```python
from build123d import *

# Parameters (mm, degrees)
EXTRUDE_2_DEPTH     = 3
SKETCH_4_R          = 2.25
SKETCH_4_R_2        = 2.5
CUT_EXTRUDE_2_DEPTH = 96.402519291
SKETCH_6_R          = 3.5
CUT_EXTRUDE_3_DEPTH = 96.402519291
SKETCH_7_R          = 3.5
CUT_EXTRUDE_4_DEPTH = 96.402519291
CUT_EXTRUDE_5_DEPTH = 96.402519291


with BuildPart() as part:
    # 草图2 → 凸台-拉伸2 (new body)
    with BuildSketch(Plane(origin=(0, 0, 0), x_dir=(1, 0, 0), z_dir=(0, 1, 0))):
        with BuildLine():
            Line((-58.569449541, 23.337085947), (32.740581269, -53.879999426))
            ThreePointArc((32.740581269, -53.879999426), (53.033008589, -53.033008589), (53.879999426, -32.740581269))
            Line((53.879999426, -32.740581269), (-23.337085947, 58.569449541))
            ThreePointArc((-23.337085947, 58.569449541), (-60.104076401, 60.104076401), (-58.569449541, 23.337085947))
        make_face()
    extrude(amount=EXTRUDE_2_DEPTH)

    # 草图4 → 切除-拉伸2 (cut, through all)
    with BuildSketch(Plane(origin=(0, 3, 0), x_dir=(1, 0, 0), z_dir=(0, 1, 0))):
        with Locations(Location((-42.426406871, 42.426406871, 0), (0, 0, 270))):
            Circle(SKETCH_4_R)
        with Locations(Location((42.426406871, -42.426406871, 0), (0, 0, 270))):
            Circle(SKETCH_4_R_2)
    extrude(amount=-CUT_EXTRUDE_2_DEPTH, mode=Mode.SUBTRACT)

    # 草图6 → 切除-拉伸3 (cut, through all)
    with BuildSketch(Plane(origin=(0, 3, 0), x_dir=(1, 0, 0), z_dir=(0, 1, 0))):
        with Locations(Location((-42.426406871, 42.426406871, 0), (0, 0, 270))):
            Circle(SKETCH_6_R)
    extrude(amount=-CUT_EXTRUDE_3_DEPTH, mode=Mode.SUBTRACT)

    # 草图7 → 切除-拉伸4 (cut, through all)
    with BuildSketch(Plane(origin=(0, 3, 0), x_dir=(1, 0, 0), z_dir=(0, 1, 0))):
        with Locations(Location((42.426406871, -42.426406871, 0), (0, 0, 270))):
            Circle(SKETCH_7_R)
    extrude(amount=-CUT_EXTRUDE_4_DEPTH, mode=Mode.SUBTRACT)

    # 草图8 → 切除-拉伸5 (cut, through all)
    with BuildSketch(Plane(origin=(0, 3, 0), x_dir=(1, 0, 0), z_dir=(0, 1, 0))):
        Polygon((33.626672858, -22.564710472), (-15.702999665, 25.870376375), (-26.891422763, 12.98046534), (25.218843822, -32.251166492), align=None)
    extrude(amount=-CUT_EXTRUDE_5_DEPTH, mode=Mode.SUBTRACT)


solid = part.part
```
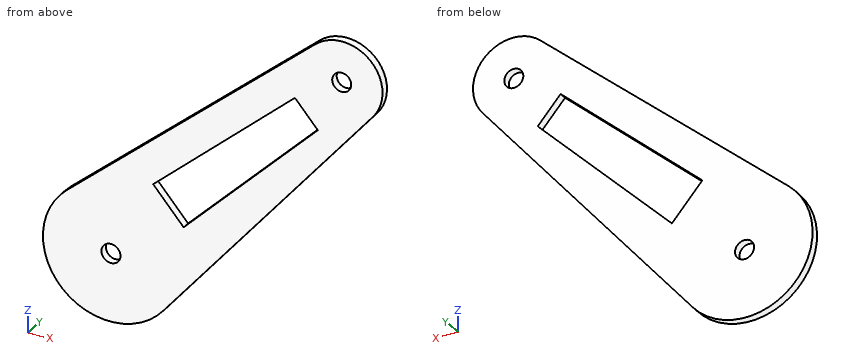
Design review of the part built by this model. Coordinates are the model's own, in mm. Round coordinates to 2 decimals unless told otherwise and drop trailing zeros. Write each loop counter-clockwise with the first axis right and the second up, starting at its lowest first coordinate (ties: lowest second). Pieces come first, ordered by that corner, then holes. Notation, with made-up numbers: (75.5, -26) -> (86.5, -26) arc R9 cw to (86.5, -10) -> close; hole circle Ø11 at (-29.5, 60.5). An arc over 180 degrees is marked (long way). Write item = value, one per line. Start each with the question number.
1) Take a section at C-C, the plane y = 1.5. State the section outline as (x, z) points, plus the area to 3 significant figures.
2) Take a section at A-A, the plane x = 30.5. State the section outline as (y, z) points, plus the area to 3 significant figures.
3) Take a section at B-B, the plane z = -21. State the section outline as (x, y) points.
4) Take a section at D-D, the plane z = -47.5. State the section outline as (x, y) points, plus the area to 3 significant figures.
5) Wall thickness on probe 1 along X at (y, z) = (2, 8); probe 2 along Z at (x, y) = (45.5, 1.9); probe 3 along Z at (x, y) = (19, 2.75): over which ranges is each line inside the solid? List them lowest first. Write a range as from..to.
Results list:
q1.outline = (-58.57, -23.34) arc R25 ccw (long way) to (-23.34, -58.57) -> (53.88, 32.74) arc R15 ccw to (32.74, 53.88) -> close; hole circle Ø7 at (-42.43, -42.43); hole (-26.89, -12.98) -> (-15.7, -25.87) -> (33.63, 22.56) -> (25.22, 32.25) -> close; hole circle Ø7 at (42.43, 42.43)
q1.area = 5,040 mm²
q2.outline = (0, 5.09) -> (3, 5.09) -> (3, 19.49) -> (0, 19.49) -> close; (0, 26.17) -> (3, 26.17) -> (3, 51.99) -> (0, 51.99) -> close
q2.area = 121 mm²
q3.outline = (-55.81, 0) -> (-19.93, 0) -> (-19.93, 3) -> (-55.81, 3) -> close; (-10.74, 0) -> (8.43, 0) -> (8.43, 3) -> (-10.74, 3) -> close
q4.outline = (-66.91, 0) -> (-13.98, 0) -> (-13.98, 3) -> (-66.91, 3) -> close
q4.area = 159 mm²
q5.probe_1 = -21.51..-2.72, 18.79..32.96
q5.probe_2 = 22.83..40.75, 44.1..57.11
q5.probe_3 = -8.51..8.2, 26.85..42.26
